```python
from build123d import *

# Parameters (mm, degrees)
F0_W     = 38.1
F0_H     = 143.9402176437
F0_H_2   = 25.2968176437
F0_W_2   = 368.3
F0_H_3   = 33.7566
F0_H_4   = 50.9031823563
F0_H_5   = 25.4
F0_H_6   = 50.8
F1_DEPTH = 25.4
F2_W     = 38.1
F2_H     = 25.4
F3_DEPTH = 203.2
F5_DEPTH = 38.1
F7_DEPTH = 38.1
F8_W     = 25.4
F8_H     = 50.8
F9_DEPTH = 25.4


with BuildPart() as f1:
    # F0 (on Front) → F1 (new body)
    with BuildSketch(Plane.XZ):
        with Locations((203.2, 16.9298911782)):
            Rectangle(F0_W, F0_H)
        with Locations((203.2, 126.9484088218)):
            Rectangle(F0_W, F0_H_2)
        with Locations((0, -71.9185176437)):
            Rectangle(F0_W_2, F0_H_3)
        with Locations((203.2, -71.9185176437)):
            Rectangle(F0_W, F0_H_3)
        with Locations((-203.2, -114.2484088218)):
            Rectangle(F0_W, F0_H_4)
        with Locations((-203.2, 16.9298911782)):
            Rectangle(F0_W, F0_H)
        with Locations((-203.2, 101.6)):
            Rectangle(F0_W, F0_H_5)
        with Locations((203.2, 101.6)):
            Rectangle(F0_W, F0_H_5)
        with Locations((-203.2, 127)):
            Rectangle(F0_W, F0_H_5)
        with Locations((-203.2, -71.9185176437)):
            Rectangle(F0_W, F0_H_3)
        with Locations((0, 101.6)):
            Rectangle(F0_W_2, F0_H_5)
        with Locations((203.2, -114.1968176437)):
            Rectangle(F0_W, F0_H_6)
    extrude(amount=F1_DEPTH)

    # F2 (on face) → F3 (join)
    with BuildSketch(Plane.XZ.offset(25.4)):
        with Locations((-203.2, 101.6)):
            Rectangle(F2_W, F2_H)
        with Locations((203.2, 101.6)):
            Rectangle(F2_W, F2_H)
    extrude(amount=F3_DEPTH)

    # F4 (on face) → F5 (join)
    with BuildSketch(Plane(origin=(-222.25, 0, 0), x_dir=(0, -1, 0), z_dir=(-1, 0, 0))):
        Polygon((25.4, -88.9), (228.6, 88.9), (190.0277566224, 88.9), (25.4, -55.1492870446), align=None)
    extrude(amount=-F5_DEPTH)

    # F6 (on face) → F7 (join)
    with BuildSketch(Plane.YZ.offset(222.25)):
        Polygon((-25.4, -55.0545965492), (-190.0150696827, 88.9), (-228.6, 88.9), (-25.4, -88.7968176437), align=None)
    extrude(amount=-F7_DEPTH)

    # F8 (on face) → F9 (join)
    with BuildSketch(Plane.XY.offset(114.3)):
        with Locations((-234.95, -254)):
            Rectangle(F8_W, F8_H)
        with Locations((-234.95, -203.2)):
            Rectangle(F8_W, F8_H)
        with Locations((234.95, -203.2)):
            Rectangle(F8_W, F8_H)
        with Locations((234.95, -254)):
            Rectangle(F8_W, F8_H)
    extrude(amount=-F9_DEPTH)


solid = f1.part
```
Source: CAD feature listing. Evaluate the final solid. Frame: model axes, mm. A direction names the side the tool comes from. Give positions to 0.01 mm unless a question says otherwise; leave off trailing zeros. Loops run counter-clockwise (first coordinate to the right, second up) from the corner with the lowest first, then second, coordinate; pieces in that order, holes last. Notation, with made-up numbers: (65.5, 88.25) - (74.5, 88.25) arc R33 ccw to (74.5, 124.25) - close; hole circle Ø3 at (15.25, 51). An arc over 180 degrees is marked (long way). Use CSV: the item, a comma, the result in double quotes.
1) Mould query, pull axis Z, two halves, no side actions, for faces 1 (the flat face through (-184.15, -13, 16)), 2 (the flat face through (235, -177.8, 102)), 3 (the flat face through (203.47, -106.56, 15.92)), 4 (the flat face through (-209, -151, 114.3)). Classes: +Z half, -Z half, draft (parallel to the pull), parting line (faces both ways), or undercut.
Worked out:
face 1,"undercut"
face 2,"draft"
face 3,"undercut"
face 4,"+Z half"
2) Set-up query: faces 5 (the flat face through (203, -25.4, -114)), 6 (the flat face through (203, -228.6, 102)), 7 (the flat face through (-3, -13, -88.797)), 8 (the flat face through (-203, -25.4, 127)). Return all of +Z, -Z, +X, -X, +Y, -Y with unobstructed straight access to the full face (end or side cutting, diameter ignored); none if empty.
Worked out:
face 5,"-Z, +X, -X, -Y"
face 6,"+Z, -Z, -Y"
face 7,"-Z, +Y, -Y"
face 8,"+Z, +X, -X, -Y"
3) Cut plane D-D (z = -9.5). Output: boundary loops of the cut face in (x, y).
Worked out:
outline,"(-222.25, -116.14) - (-184.15, -116.14) - (-184.15, -77.57) - (-222.25, -77.57) - close; (-222.25, -25.4) - (-184.15, -25.4) - (-184.15, 0) - (-222.25, 0) - close; (184.15, -116.08) - (222.25, -116.08) - (222.25, -77.49) - (184.15, -77.49) - close; (184.15, -25.4) - (222.25, -25.4) - (222.25, 0) - (184.15, 0) - close"
4) Pin query (flat end, axial travel): P1, Ø12.5, axis at x = -199.5, z = 106, coming from the -Y side; P2, Ø7.5, axis at x = -66, y = -8.5, coming from the -Z side; P3, Ø7.5, axis at y = -9.5, z = -121, coming from the -X side; P4, Ø1, axis at x = 54, z = 87, coming from the +Y side. Return the tip coordinate at first contact, or that it passes through.
Worked out:
P1,"stops at y = -228.6"
P2,"stops at z = -88.8"
P3,"stops at x = -222.25"
P4,"passes through"
5) Line query: line 1 (X direction, y = -188, z = 55); line 2 (Y direction, x = 185, z = 50). Output: solid intervals per line, ascending.
Worked out:
line 1,"x = -222.25 to -184.15, 184.15 to 222.25"
line 2,"y = -184.12 to -145.53, -25.4 to 0"
6) Cut plane B-B (x = 75). Output: boundary loops of the cut face in (y, z), and give its area (3 significant figures).
Worked out:
outline,"(-25.4, -88.8) - (0, -88.8) - (0, -55.04) - (-25.4, -55.04) - close; (-25.4, 88.9) - (0, 88.9) - (0, 114.3) - (-25.4, 114.3) - close"
area,"1,500 mm^2"
7) Cut plane A-A (z = -117.5). Output: boundary loops of the cut face in (x, y).
Worked out:
outline,"(-222.25, -25.4) - (-184.15, -25.4) - (-184.15, 0) - (-222.25, 0) - close; (184.15, -25.4) - (222.25, -25.4) - (222.25, 0) - (184.15, 0) - close"
8) Cut plane C-C (y = -16.5). Output: boundary loops of the cut face in (x, z), and give its area (3 significant figures).
Worked out:
outline,"(-222.25, -139.7) - (-184.15, -139.7) - (-184.15, -88.8) - (184.15, -88.8) - (184.15, -139.6) - (222.25, -139.6) - (222.25, 139.6) - (184.15, 139.6) - (184.15, 114.3) - (-184.15, 114.3) - (-184.15, 139.7) - (-222.25, 139.7) - close; hole (-184.15, -55.04) - (184.15, -55.04) - (184.15, 88.9) - (-184.15, 88.9) - close"
area,"43,100 mm^2"
